Source: CAD feature listing. Evaluate the final solid. Frame: model axes, mm. A direction names the side the tool comes from. Give positions to 0.01 mm unless a question says otherwise; leave off trailing zeros. Write each loop counter-clockwise with the first axis right and the second up, starting at its lowest first coordinate (ties: lowest second). Pieces come first, ordered by that corner, then holes. Notation, with made-up numbers: M -22.5,48 L 20.5,48 A10 cw 20.5,64 Z; hole C 77.5,71.5 d5. An arc over 180 degrees is marked long. Answer as a JSON object with one key per item and string values. Group by question number.
```python
from build123d import *

# Parameters (mm, degrees)
SKETCH_4_R          = 4
CUT_EXTRUDE_1_DEPTH = 4.7
HOLE_WIZARD_M5_1_D  = 4.2


with BuildPart() as part:
    # 草图1 → 旋转1 (revolve)
    with BuildSketch(Plane.XY, mode=Mode.PRIVATE) as revolve_1_sk:
        Polygon((24, 12.2), (24, 6), (19, 6), (19, 0), (19, -1), (16, -1), (16, 0), (16, 3), (15, 3), (15, 8.5), (16, 8.5), (16, 12.5), (17.5, 12.5), (17.5, 17.2), (21.5, 17.2), (40, 17.2), (40, 12.2), align=None)
    revolve(revolve_1_sk.sketch.rotate(Axis((0, 0, 0), (0, 1, 0)), 90), axis=Axis((0, 0, 0), (0, 1, 0)))

    # 草图4 → 切除-拉伸1 (cut)
    with BuildSketch(Plane(origin=(0, 17.2, 0), x_dir=(1, 0, 0), z_dir=(0, 1, 0))):
        with Locations((0, -17.5)):
            Circle(SKETCH_4_R)
        with Locations((17.5, 0)):
            Circle(SKETCH_4_R)
        with Locations((0, 17.5)):
            Circle(SKETCH_4_R)
        with Locations((-17.5, 0)):
            Circle(SKETCH_4_R)
    extrude(amount=-CUT_EXTRUDE_1_DEPTH, mode=Mode.SUBTRACT)

    # M5 螺纹孔1 (through all)
    with Locations(Plane(origin=(17.5, 17.2, -30.310889132), x_dir=(0, 0, 1), z_dir=(0, 1, 0))):
        with Locations((0, 0), (30.310889132, 17.5), (60.621778264, 0), (60.621778264, -35), (30.310889132, -52.5), (0, -35)):
            Hole(HOLE_WIZARD_M5_1_D / 2)


solid = part.part
```
(1) Section D-D, the plane z = -20.5. Return loops of the section in (x, y), plus the area to 3 significant figures.
(2) Section A-A, the plane x = 0. Return loops of the section in (y, z).
(3) Section C-C, the plane z = -10.5. Return loops of the section in (x, y), plus the area to 3 significant figures.
(4) Access query for faces 1 (the cylindrical face through (15.62, 10.53, 3.47)), 2 (the cylindrical face through (15.62, 0.97, 3.47)), 3 (the flat face through (17, 17.2, -8)). Directions: +Z, -Z, +X, -X, +Y, -Y. A direction counts if a zero-diameter tool reaches every point of the face in a straight line with its end or side. Return the directions, or none.
(5) Contact query for flat-ended pins moving along their axis: pin 1 Ø1.5 at (x, y) = (-4.5, 12.5) entering from -Z; pin 2 Ø2 at (y, z) = (10, 7.5) entering from -X; pin 3 Ø6.5 at (x, z) = (17.5, 0) entering from +Y. Output: stop coordinate, or through.
(6) Section B-B, the plane z = 0. State how many separate pieces and enclosed holes the cut face has, plus the area to 4 significant figures.
(7) Ray query, L1, parallel to X at y = 15.1, z = 0; L2, parallel to X at y = 13, z = 30.5; L3, parallel to X at y = 14.5, z = -31. Return the intervals inside material, ascending. Write a range as [from, to].
Reported:
{
 "1": {"outline": "M -34.35,12.2 L -12.48,12.2 L -12.48,6 L 12.48,6 L 12.48,12.2 L 34.35,12.2 L 34.35,17.2 L 2.65,17.2 L 2.65,12.5 L -2.65,12.5 L -2.65,17.2 L -34.35,17.2 Z", "area": "473 mm2"},
 "2": {"outline": "M -1,-19 L 6,-19 L 6,-24 L 12.2,-24 L 12.2,-40 L 17.2,-40 L 17.2,-21.5 L 12.5,-21.5 L 12.5,-16 L 8.5,-16 L 8.5,-15 L 3,-15 L 3,-16 L -1,-16 Z; M -1,16 L 3,16 L 3,15 L 8.5,15 L 8.5,16 L 12.5,16 L 12.5,21.5 L 17.2,21.5 L 17.2,40 L 12.2,40 L 12.2,24 L 6,24 L 6,19 L -1,19 Z"},
 "3": {"outline": "M -38.6,12.2 L -21.58,12.2 L -21.58,6 L -15.84,6 L -15.84,-1 L -12.07,-1 L -12.07,3 L -10.71,3 L -10.71,8.5 L -12.07,8.5 L -12.07,12.5 L -14,12.5 L -14,17.2 L -38.6,17.2 Z; M 10.71,3 L 12.07,3 L 12.07,-1 L 15.84,-1 L 15.84,6 L 21.58,6 L 21.58,12.2 L 38.6,12.2 L 38.6,17.2 L 14,17.2 L 14,12.5 L 12.07,12.5 L 12.07,8.5 L 10.71,8.5 Z", "area": "433 mm2"},
 "4": {"face 1": "+Y", "face 2": "-Y", "face 3": "+Z, -Z, +X, -X, +Y"},
 "5": {"pin 1": "stops at z = -39.82", "pin 2": "stops at x = -23.1", "pin 3": "stops at y = 12.5"},
 "6": {"separate pieces": "4", "enclosed holes": "0", "area": "298.5 mm2"},
 "7": {"L1": "x = [-40, -37.1], [-32.9, -21.5], [21.5, 32.9], [37.1, 40]", "L2": "x = [-25.88, -19.59], [-15.41, 15.41], [19.59, 25.88]", "L3": "x = [-25.28, -19.48], [-15.52, 15.52], [19.48, 25.28]"}
}
